```python
from build123d import *

# Parameters (mm, degrees)
BRIDA_BASE1_DEPTH                = 50.8
CROQUIS8_W                       = 6.35
CROQUIS8_H                       = 12.7
CORTAR_EXTRUIR2_DEPTH            = 56.160268355
MATRIZL1_COUNT                   = 2
MATRIZL1_PITCH                   = 25.4
BRIDA_DE_ARISTA1_STRIP_W         = 6.7564
BRIDA_DE_ARISTA1_STRIP_H         = 1.524
BRIDA_DE_ARISTA1_STRIP_CUT_DEPTH = 50.8
BRIDA_DE_ARISTA1_DEPTH           = 50.8


# Sheet-metal steps are written as plain solids
with BuildPart() as part:
    # Croquis1 → Brida base1 (new body)
    with BuildSketch(Plane.XY):
        with BuildLine():
            Line((0, 0), (-17.4625, 0))
            ThreePointArc((-17.4625, 0), (-18.562352263, 2.73226253), (-15.876270508, 1.524))
            Line((-15.876270508, 1.524), (-14.353490196, 1.46304))
            ThreePointArc((-14.353490196, 1.46304), (-19.618210435, 3.831234559), (-17.4625, -1.524))
            Line((-17.4625, -1.524), (0, -1.524))
            Line((0, -1.524), (0, 0))
        make_face()
    extrude(amount=BRIDA_BASE1_DEPTH)

    # Croquis8 → Cortar-Extruir2 (cut, through all)
    with BuildSketch(Plane.XZ.offset(1.524)):
        with Locations((-17.399, 44.45)):
            Rectangle(CROQUIS8_W, CROQUIS8_H)
    cortar_extruir2 = extrude(amount=-CORTAR_EXTRUIR2_DEPTH, mode=Mode.SUBTRACT)

    # MatrizL1: Cortar-Extruir2 ×2
    with Locations(*[(0, 0, -i * MATRIZL1_PITCH) for i in range(1, MATRIZL1_COUNT)]):
        add(cortar_extruir2, mode=Mode.SUBTRACT)

    # Brida de arista1 strip (across the edge) → Brida de arista1 strip cut (cut)
    with BuildSketch(Plane(origin=(0, -1.524, 0), x_dir=(-1, 0, 0), z_dir=(0, 0, 1))):
        with Locations((-1.524, -0.762)):
            Rectangle(BRIDA_DE_ARISTA1_STRIP_W, BRIDA_DE_ARISTA1_STRIP_H)
    extrude(amount=BRIDA_DE_ARISTA1_STRIP_CUT_DEPTH, mode=Mode.SUBTRACT)

    # Brida de arista1 section (across the edge) → Brida de arista1 (add)
    with BuildSketch(Plane(origin=(0, -1.524, 0), x_dir=(-1, 0, 0), z_dir=(0, 0, 1))):
        with BuildLine():
            Line((0, 0.3302), (0, 17.526))
            Line((0, 17.526), (1.524, 17.526))
            Line((1.524, 17.526), (1.524, 0.3302))
            ThreePointArc((1.524, 0.3302), (1.620713341, 0.096713341), (1.8542, 0))
            Line((1.8542, 0), (1.8542, -1.524))
            ThreePointArc((1.8542, -1.524), (0.543082606, -0.980917394), (0, 0.3302))
        make_face()
    extrude(amount=BRIDA_DE_ARISTA1_DEPTH)


solid = part.part
```
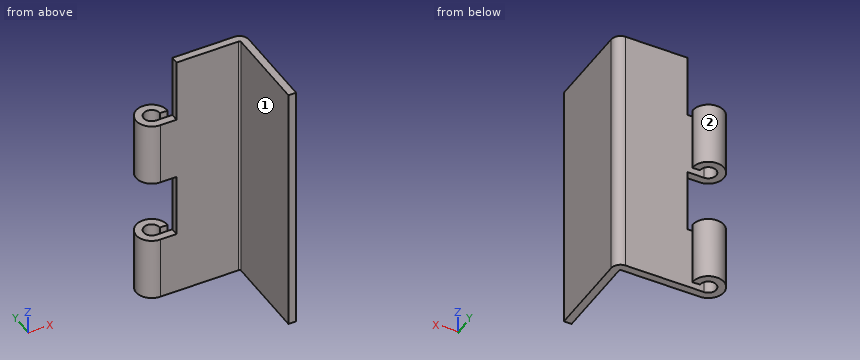
Check sheet for the modelled part. Datum: model origin and axes. Units: mm. Face numbers are marked on the shaded views. A direction names the side the tool comes from. Round coordinates to 2 decimals unless told otherwise and drop trailing zeros. Loops run counter-clockwise (first coordinate to the right, second up) from the corner with the lowest first, then second, coordinate; pieces in that order, holes last. Notation, with made-up numbers: (-9.5, 12.25) -> (23.5, 12.25) arc R17 ccw to (23.5, 39.25) -> close; hole circle Ø3 at (43.5, 7.25). An arc over 180 degrees is marked (long way). Write item = value, one per line. Start each with the question number.
1) Sectioned sample at B-B, the plane x = -8.75. Record the cut outline in (y, z).
2) Thickness scan on probe 1 along Z at (x, y) = (-19, 3); probe 2 along X at (y, z) = (-10.25, 38). Record the ranges inside material, lowest first.
3) Gauge pin test, flat ends, axial feed: pin 1 Ø10 at (x, z) = (-4.5, 13) entering from +Y; pin 2 Ø6 at (y, z) = (-9, 18) entering from -X; pin 3 Ø1.9 at (x, y) = (-18, 1) entering from +Z. Record the tip position at first contact, or that the pin passes through.
4) Set-up check for the marked faces 1 and 2: record each of +Z, -Z, +X, -X, +Y, -Y from which the full face is reachable in a straight line by a thin tool's end or side.
5) Sectioned sample at C-C, the plane z = 41.5. Record the cut outline in (x, y).
Results are:
q1.outline = (-1.52, 0) -> (0, 0) -> (0, 50.8) -> (-1.52, 50.8) -> close
q2.probe_1 = 0 to 12.7, 25.4 to 38.1
q2.probe_2 = -1.52 to 0
q3.pin_1 = 0
q3.pin_2 = -1.52
q3.pin_3 = 38.1
q4.face_1 = +Z, -Z, -X, -Y
q4.face_2 = +Z, -Z
q5.outline = (-14.22, -1.52) -> (-1.85, -1.52) arc R0.33 cw to (-1.52, -1.85) -> (-1.52, -19.05) -> (0, -19.05) -> (0, -1.85) arc R1.85 ccw to (-1.85, 0) -> (-14.22, 0) -> close
